Geometry: final body of the model. Coordinates: model frame, mm. A direction names the side the tool comes from. Round coordinates to 2 decimals unless told otherwise and drop trailing zeros. Order: outer loops, then holes, each group sorted by start corner. A loop starts at its lowest first (then second) coordinate and runs counter-clockwise, first axis right, second up. Notation, with made-up numbers: M -39,-38.75 L 5,-38.75 A15 cw 5,-27.75 Z; hole C -33,16.25 d8. An arc over 180 degrees is marked long. Return JSON: item names as keys, results as strings. Group by question number.
Q1. Ray query, probe 1 along Y at (x, z) = (38.5, 39); probe 2 along Y at (x, z) = (-14.5, 51); probe 3 along X at (y, z) = (-22, 2.5) (3 decimals). Return the intervals inside material, ascending.
Q2. Mould query, pull axis X, two halves, no side actions, for faces 1 (the face through (39.464, 61.59, 0.133)), 2 (the face through (45.8, -0.4, 38.1)), 3 (the face through (-39.464, 61.59, -0.133)), 4 (the face through (45, -25.4, 42)). Classes: released by +X, released by -X, zero draft, split by the parting line, or undercut.
Q3. Contact query for flat-ended pins moving along their axis: pin 1 (12.5 mm diameter, centred on x = 64, y = 5.5, fed in from -Z); pin 2 (1.5 mm diameter, centred on x = -5, y = -49.5, fed in from +Z) (3 decimals); pin 3 (19 mm diameter, centred on y = -18, z = 14.5, fed in from -X) (3 decimals); pin 4 (4 mm diameter, centred on y = 7, z = -2, fed in from +X) (3 decimals). Output: stop coordinate, or through.
Q4. Cut plane B-B on y = -29. Output: boundary loops of the cut face in (x, z) (3 decimals).
Q5. Cut plane A-A on z = -4. Output: boundary loops of the cut face in (x, y) (3 decimals), and give its area (3 significant figures).
Q6. Access query for faces 5 (the face through (81.422, 0.962, 38.078)), 6 (the face through (41.275, -1, 4)), 7 (the face through (22.225, 17, 18)), 8 (the face through (32.65, -16.79, 51.89)). Directions: +Z, -Z, +X, -X, +Y, -Y. A direction counts if a zero-diameter tool reaches every point of the face in a straight line with its end or side. Return the directions, or none.
```python
from build123d import *

# Parameters (mm, degrees)
F1_DEPTH = 63.5
F2_DEPTH = 25.4
F3_DEPTH = 7.9375
F5_R     = 6.35


with BuildPart() as f1:
    # F0 (on Front) → F1 (new body, symmetric)
    with BuildSketch(Plane.XZ):
        Polygon((41.275, -9.525), (41.275, 9.525), (22.225, 9.525), (-41.275, 9.525), (-41.275, -9.525), align=None)
    extrude(amount=F1_DEPTH, both=True)

    # F0 (on Front) → F2 (join, symmetric)
    with BuildSketch(Plane.XZ):
        with BuildLine():
            Line((22.225, 9.525), (41.275, 9.525))
            Line((41.275, 9.525), (41.275, 27.0002))
            ThreePointArc((41.275, 27.0002), (45.9246798487, 38.2255201513), (57.15, 42.8752))
            Line((57.15, 42.8752), (57.15, 61.9252))
            add(Edge.make_bspline(
                [(56.9266506974, 61.9244858207), (57.001194094, 61.9246904131), (57.0756440835, 61.9249282445), (57.15, 61.9252)],
                knots=[111.2718154364, 111.2718154364, 111.2718154364, 111.2718154364, 111.5045361635, 111.5045361635, 111.5045361635, 111.5045361635], degree=3))
            ThreePointArc((56.9266506974, 61.9244858207), (32.3754556107, 51.6168117754), (22.225, 27.0002))
            Line((22.225, 27.0002), (22.225, 9.525))
        make_face()
        Polygon((57.15, 61.9252), (57.15, 42.8752), (82.639603816, 42.8752), (82.4913637761, 61.9252), align=None)
    extrude(amount=F2_DEPTH, both=True)

    # F0 (on Front) → F3 (join, symmetric)
    with BuildSketch(Plane.XZ):
        with BuildLine():
            Line((-41.275, 9.525), (22.225, 9.525))
            Line((22.225, 9.525), (22.225, 27.0002))
            ThreePointArc((22.225, 27.0002), (32.3754556107, 51.6168117754), (56.9266506974, 61.9244858207))
            add(Edge.make_bspline(
                [(-41.275, 9.525), (-35.7109377895, 69.3276862996), (21.2848788051, 61.8266631405), (56.9266506974, 61.9244858207)],
                knots=[0, 0, 0, 0, 111.2718154364, 111.2718154364, 111.2718154364, 111.2718154364], degree=3))
        make_face()
    extrude(amount=F3_DEPTH, both=True)

    # F0 (on Front) → F4 (revolve)
    with BuildSketch(Plane.XZ):
        Polygon((82.4913637761, 61.9252), (82.639603816, 42.8752), (82.6767626526, 38.1), (107.95, 38.1), (107.95, 66.675), (82.4544025928, 66.675), align=None)
    revolve(axis=Axis((82.5655826227, 0, 52.3875), (0.0077813938, 0, -0.9999697245)))

    # F5
    f5_edges = [f1.edges().sort_by_distance(p)[0] for p in [
        (41.275, -63.5, 0),
        (-41.275, -63.5, 0),
        (41.275, 63.5, 0),
        (-41.275, 63.5, 0),
    ]]
    fillet(f5_edges, radius=F5_R)


solid = f1.part
```
Result sheet:
{
 "1": {"probe 1": "y = -25.4 to 25.4", "probe 2": "y = -7.94 to 7.94", "probe 3": "x = -41.275 to 41.275"},
 "2": {"face 1": "released by +X", "face 2": "undercut", "face 3": "released by -X", "face 4": "zero draft"},
 "3": {"pin 1": "stops at z = 37.71", "pin 2": "stops at z = 9.525", "pin 3": "stops at x = -41.275", "pin 4": "stops at x = 41.275"},
 "4": {"outline": "M -41.275,-9.525 L 41.275,-9.525 L 41.275,9.525 L -41.275,9.525 Z"},
 "5": {"outline": "M -41.275,-57.15 A6.35 ccw -34.925,-63.5 L 34.925,-63.5 A6.35 ccw 41.275,-57.15 L 41.275,57.15 A6.35 ccw 34.925,63.5 L -34.925,63.5 A6.35 ccw -41.275,57.15 Z", "area": "10,400 mm²"},
 "6": {"face 5": "-Z, +X", "face 6": "-Z, +X, +Y, -Y", "face 7": "+Z, -X, +Y", "face 8": "+Z, -X, -Y"}
}
